Verification items for the finished model (mm, model axes). Give positions to 0.01 mm unless a question says otherwise; leave off trailing zeros. Write each loop counter-clockwise with the first axis right and the second up, starting at its lowest first coordinate (ties: lowest second). Pieces come first, ordered by that corner, then holes. Notation, with made-up numbers: (-29.5, 61.25) - (-9.5, 61.25) arc R30 ccw to (-9.5, 86.25) - close; hole circle Ø3 at (83.5, 72.25). An arc over 180 degrees is marked (long way). Put each result on its own line as item: value.
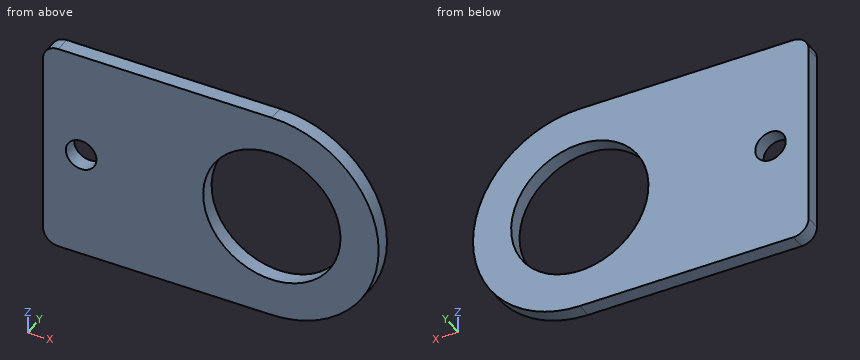
from build123d import *

# Parameters (mm, degrees)
SKETCH1_R           = 2
SKETCH1_R_2         = 9
BOSS_EXTRUDE1_DEPTH = 2
FILLET1_R           = 2


with BuildPart() as part:
    # Sketch1 → Boss-Extrude1 (new body)
    with BuildSketch(Plane(origin=(0, 0, 0), x_dir=(1, 0, 0), z_dir=(0, 1, 0))):
        with BuildLine():
            Line((-15, -14), (15, -14))
            ThreePointArc((15, -14), (29, 0), (15, 14))
            Line((15, 14), (-15, 14))
            Line((-15, 14), (-15, -14))
        make_face()
        with Locations(Location((-10, 0, 0), (0, 0, 270))):
            Circle(SKETCH1_R, mode=Mode.SUBTRACT)
        with Locations(Location((15, 0, 0), (0, 0, 270))):
            Circle(SKETCH1_R_2, mode=Mode.SUBTRACT)
    extrude(amount=BOSS_EXTRUDE1_DEPTH)

    # Fillet1
    fillet1_edges = [part.edges().sort_by_distance(p)[0] for p in [
        (-15, 1, 14),
        (-15, 1, -14),
    ]]
    fillet(fillet1_edges, radius=FILLET1_R)


solid = part.part
Q1. Go/stop test with a flat-tipped pin: pin 1 Ø16 at (x, z) = (15, 0) entering from -Y. Record where the tip stops, or that it passes through.
Answers follow:
pin 1: passes through
Q2. Section check C-C, the plane z = 0. Record the cut outline in (x, y).
Answers follow:
outline: (-15, 0) - (-12, 0) - (-12, 2) - (-15, 2) - close; (-8, 0) - (6, 0) - (6, 2) - (-8, 2) - close; (24, 0) - (29, 0) - (29, 2) - (24, 2) - close
Q3. Scan lines: line 1 along X through (y, z) = (0.4, 0); line 2 along Z through (x, y) = (21, 0.2); line 3 along Z through (x, y) = (18, 0.8). Record each from-to range of solid material in increasing order.
Answers follow:
line 1: x = -15 to -12, -8 to 6, 24 to 29
line 2: z = -12.65 to -6.71, 6.71 to 12.65
line 3: z = -13.67 to -8.49, 8.49 to 13.67
Q4. Section check D-D, the plane z = -6.75. Record the cut outline in (x, y).
Answers follow:
outline: (-15, 0) - (9.05, 0) - (9.05, 2) - (-15, 2) - close; (20.95, 0) - (27.27, 0) - (27.27, 2) - (20.95, 2) - close
Q5. Section check A-A, the plane x = -10. Record the cut outline in (y, z), plus the area to 3 significant figures.
Answers follow:
outline: (0, -14) - (2, -14) - (2, -2) - (0, -2) - close; (0, 2) - (2, 2) - (2, 14) - (0, 14) - close
area: 48.0 mm2
Q6. Section check B-B, the plane y = 0.55. Record the cut outline in (x, z).
Answers follow:
outline: (-15, -12) arc R2 ccw to (-13, -14) - (15, -14) arc R14 ccw to (15, 14) - (-13, 14) arc R2 ccw to (-15, 12) - close; hole circle Ø4 at (-10, 0); hole circle Ø18 at (15, 0)
